Answer from the drawing. Dimensions are ordinates in mm from the lowest x, y and z of the part. A direction names the side the tool comes from. Round coordinates to 2 decimals unless told otherwise and drop trailing zeros. Loops run counter-clockwise (first coordinate to the right, second up) from the corner with the lowest first, then second, coordinate; pieces in that order, holes last. Notation, with made-up numbers: (-3, -18.5) -> (41, -18.5) arc R21 cw to (41, 5.5) -> close; hole circle Ø11 at (21.5, -28). An arc over 180 degrees is marked (long way). One line per question, with ' | ' between items.
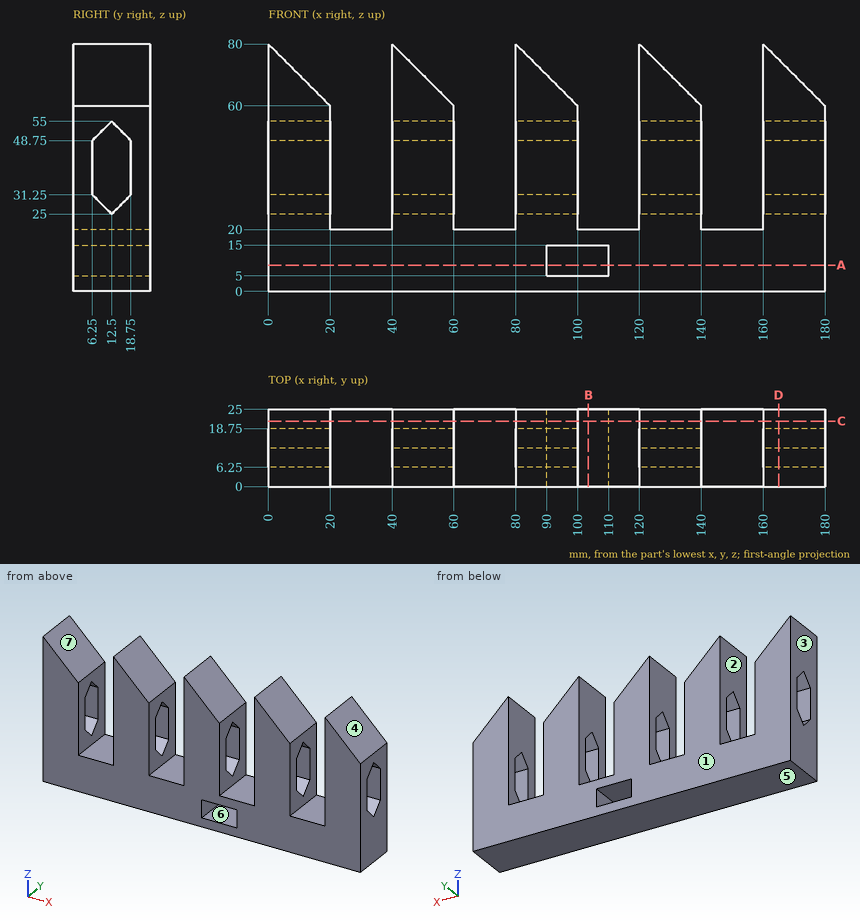
Q1. A cutting plane is placed at B-B on x = 103.5. Give the vertices of the cut face in (y, z).
Numbers:
outline: (0, 0) -> (25, 0) -> (25, 5) -> (0, 5) -> close; (0, 15) -> (25, 15) -> (25, 20) -> (0, 20) -> close
Q2. Find the intervals of material crossed by line 1 (X direction, y = 16.25, z = 63); line 2 (X direction, y = 2.5, z = 36.5); line 3 (Y direction, x = 127, z = 37), in increasing order. Write a range as from..to.
Numbers:
line 1: 0..17, 40..57, 80..97, 120..137, 160..177 | line 2: 0..20, 40..60, 80..100, 120..140, 160..180 | line 3: 0..6.25, 18.75..25
Q3. A cutting plane is placed at A-A on z = 8.5. Give the vertices of the cut face in (x, y).
Numbers:
outline: (0, 0) -> (90, 0) -> (90, 25) -> (0, 25) -> close; (110, 0) -> (180, 0) -> (180, 25) -> (110, 25) -> close
Q4. Given pin 1 Ø7.5 at (y, z) = (16.5, 46) entering from +X, flat-ended and moving along its own axis, determine where the tip first touches the part or whether it passes through.
Numbers:
pin 1: x = 180
Q5. A cutting plane is placed at D-D on x = 165. Give the vertices of the cut face in (y, z).
Numbers:
outline: (0, 0) -> (25, 0) -> (25, 75) -> (0, 75) -> close; hole (6.25, 31.25) -> (12.5, 25) -> (18.75, 31.25) -> (18.75, 48.75) -> (12.5, 55) -> (6.25, 48.75) -> close
Q6. For a pull along X with two mould halves and no side action, classify the marked faces 1, 2, 3 and 4 as pulls with the +X half, pulls with the -X half, needs draft (parallel to the pull), parting line crosses it, or undercut.
Numbers:
face 1: needs draft | face 2: undercut | face 3: pulls with the -X half | face 4: pulls with the +X half
Q7. For the marked faces 5, 6 and 7, determine the directions among +Z, -Z, +X, -X, +Y, -Y from which every point of the face is accessible in a straight line to the end or side of a thin tool.
Numbers:
face 5: -Z, +X, -X, +Y, -Y | face 6: +Y, -Y | face 7: +Z, +Y, -Y
Q8. A cutting plane is placed at C-C on y = 21.25. Give the vertices of the cut face in (x, z), plus the area to 3 significant figures.
Numbers:
outline: (0, 0) -> (180, 0) -> (180, 60) -> (160, 80) -> (160, 20) -> (140, 20) -> (140, 60) -> (120, 80) -> (120, 20) -> (100, 20) -> (100, 60) -> (80, 80) -> (80, 20) -> (60, 20) -> (60, 60) -> (40, 80) -> (40, 20) -> (20, 20) -> (20, 60) -> (0, 80) -> close; hole (90, 5) -> (110, 5) -> (110, 15) -> (90, 15) -> close | area: 8,400 mm^2
